Geometry: final body of the model. Coordinates: model frame, mm. Face numbers are marked on the shaded views. A direction names the side the tool comes from. Coordinates: 2 decimals unless noted, no trailing zeros. Order: outer loops, then holes, each group sorted by start corner. A loop starts at its lowest first (then second) coordinate and runs counter-clockwise, first axis right, second up. Notation, with made-up numbers: (82.25, 76.5) - (115.25, 76.5) arc R27 cw to (115.25, 103.5) - close; hole circle Ø11 at (30, 39.25). An arc over 180 degrees is marked (long way). Use a Markdown table: item, result. Add a question column.
```python
from build123d import *

# Parameters (mm, degrees)
SKETCH_1_R           = 25
EXTRUDE_1_DEPTH      = 500
EXTRUDE_2_DEPTH      = 5
EXTRUDE_2_DEPTH_BACK = 5


with BuildPart() as part:
    # Sketch 1 → Extrude 1 (new body)
    with BuildSketch(Plane(origin=(0, 0, 0), x_dir=(1, 0, 0), z_dir=(0, 1, 0))):
        Circle(SKETCH_1_R)
    extrude(amount=EXTRUDE_1_DEPTH)

    # Sketch 2 → Extrude 2 (add, two sides)
    with BuildSketch(Plane.XY) as extrude_2_sk:
        Polygon((-4.904147501, 415.869728805), (-126.476794097, 476.563858447), (-14.845338431, 359.271534235), (-133.474875453, 375.696686665), (-91.053404274, 339.123990271), (-221.536557101, 410.673201002), (-156.294980688, 332.640319032), (-52.729774464, 304.574199064), (-25, 275.438238439), (55.079469547, 275.438238439), (136.510624595, 343.521036234), (84.009054298, 323.576399455), (134.080402497, 381.655252369), (63.084510335, 359.271534235), (176.005774191, 480.837199539), (95.795047071, 413.774774694), (111.692244322, 528.591191642), (46.07245174, 440.657183354), align=None)
    extrude(amount=EXTRUDE_2_DEPTH)
    extrude(extrude_2_sk.sketch, amount=-EXTRUDE_2_DEPTH_BACK)


solid = part.part
```
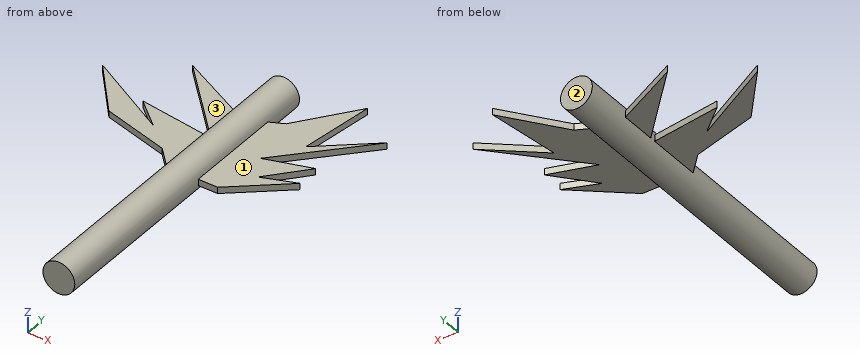
1) Set-up query: the marked faces 1, 2 and 3. Return all of +Z, -Z, +X, -X, +Y, -Y with unobstructed straight access to the full face (end or side cutting, diameter ignored); none if empty.
2) Pin query (flat end, axial travel): pin 1 (1 mm diameter, centred on y = 271.5, z = -15, fed in from +X); pin 2 (4 mm diameter, centred on y = 256, z = 0.5, fed in from -X); pin 3 (6 mm diameter, centred on y = 338.5, z = 14, fed in from +X); pin 4 (0.6 mm diameter, centred on x = -24.5, z = 3, fed in from -Y). Return the tip coordinate at first contact, or that it passes through.
3) Ray query, line 1 along Y through (x, z) = (88, -4); line 2 along Y through (x, z) = (94, -4); line 3 along Y through (x, z) = (15.5, 1.5). Return the intervals inside material, ascending.
4) Section C-C (y = 171). Return loops of the section in (x, z), then the cut area to 3 significant figures.
5) Section D-D (x = -108.5). Return loops of the section in (y, z), then the cut area to 3 significant figures.
6) Section A-A (x = 118). Return loops of the section in (y, z), then the cut area to 3 significant figures.
7) Section B-B (x = -37). Return loops of the section in (y, z), then the cut area to 3 significant figures.
Values follow:
| question | item | result |
|---|---|---|
| 1 | face 1 | +Z, +X, +Y, -Y |
| 1 | face 2 | +Z, -Z, -X, +Y |
| 1 | face 3 | +Z, -X, +Y, -Y |
| 2 | pin 1 | stops at x = 20.37 |
| 2 | pin 2 | stops at x = -25 |
| 2 | pin 3 | stops at x = 22.45 |
| 2 | pin 4 | stops at y = 0 |
| 3 | line 1 | y = 302.96 to 325.09, 328.21 to 367.13, 386.09 to 496.84 |
| 3 | line 2 | y = 307.98 to 327.37, 335.17 to 369.02, 392.55 to 504.88 |
| 3 | line 3 | y = 0 to 500 |
| 4 | outline | circle Ø50 at (0, 0) |
| 4 | area | 1,960 mm² |
| 5 | outline | (319.69, -5) - (348.69, -5) - (348.69, 5) - (319.69, 5) - close; (354.17, -5) - (372.24, -5) - (372.24, 5) - (354.17, 5) - close; (457.68, -5) - (467.59, -5) - (467.59, 5) - (457.68, 5) - close |
| 5 | area | 570 mm² |
| 6 | outline | (328.04, -5) - (336.49, -5) - (336.49, 5) - (328.04, 5) - close; (363, -5) - (376.59, -5) - (376.59, 5) - (363, 5) - close; (418.39, -5) - (432.34, -5) - (432.34, 5) - (418.39, 5) - close |
| 6 | area | 360 mm² |
| 7 | outline | (288.05, -5) - (362.34, -5) - (362.34, 5) - (288.05, 5) - close; (382.55, -5) - (431.89, -5) - (431.89, 5) - (382.55, 5) - close |
| 7 | area | 1,240 mm² |
